from build123d import *

# Parameters (mm, degrees)
SKETCH1_W           = 78.9
SKETCH1_H           = 113.78
SKETCH1_R           = 2.75
BOSS_EXTRUDE1_DEPTH = 10
SKETCH2_R           = 11
CUT_EXTRUDE1_DEPTH  = 10
SKETCH3_R           = 22
CUT_EXTRUDE2_DEPTH  = 3
FILLET1_R           = 10


with BuildPart() as part:
    # Sketch1 → Boss-Extrude1 (new body)
    with BuildSketch(Plane(origin=(0, 0, 0), x_dir=(1, 0, 0), z_dir=(0, 1, 0))):
        with Locations((29.45, 46.89)):
            Rectangle(SKETCH1_W, SKETCH1_H)
        with Locations(Location((0, 93.78, 0), (0, 0, 270))):
            Circle(SKETCH1_R, mode=Mode.SUBTRACT)
        with Locations(Location((58.9, 93.78, 0), (0, 0, 270))):
            Circle(SKETCH1_R, mode=Mode.SUBTRACT)
        with Locations(Location((58.9, 0, 0), (0, 0, 270))):
            Circle(SKETCH1_R, mode=Mode.SUBTRACT)
        with Locations(Location((0, 0, 0), (0, 0, 270))):
            Circle(SKETCH1_R, mode=Mode.SUBTRACT)
        with Locations(Location((5.88, 70.46, 0), (0, 0, 270))):
            Circle(SKETCH1_R, mode=Mode.SUBTRACT)
        with Locations(Location((53.02, 70.46, 0), (0, 0, 270))):
            Circle(SKETCH1_R, mode=Mode.SUBTRACT)
        with Locations(Location((53.02, 23.32, 0), (0, 0, 270))):
            Circle(SKETCH1_R, mode=Mode.SUBTRACT)
        with Locations(Location((5.88, 23.32, 0), (0, 0, 270))):
            Circle(SKETCH1_R, mode=Mode.SUBTRACT)
    extrude(amount=BOSS_EXTRUDE1_DEPTH)

    # Sketch2 → Cut-Extrude1 (cut)
    with BuildSketch(Plane(origin=(0, 10, 0), x_dir=(1, 0, 0), z_dir=(0, 1, 0))):
        with Locations(Location((29.45, 46.89, 0), (0, 0, 270))):
            Circle(SKETCH2_R)
    extrude(amount=-CUT_EXTRUDE1_DEPTH, mode=Mode.SUBTRACT)

    # Sketch3 → Cut-Extrude2 (cut)
    with BuildSketch(Plane(origin=(0, 10, 0), x_dir=(1, 0, 0), z_dir=(0, 1, 0))):
        with Locations(Location((29.45, 46.89, 0), (0, 0, 270))):
            Circle(SKETCH3_R)
    extrude(amount=-CUT_EXTRUDE2_DEPTH, mode=Mode.SUBTRACT)

    # Fillet1
    fillet1_edges = [part.edges().sort_by_distance(p)[0] for p in [
        (-10, 5, 10),
        (-10, 5, -103.78),
        (68.9, 5, -103.78),
        (68.9, 5, 10),
    ]]
    fillet(fillet1_edges, radius=FILLET1_R)


solid = part.part
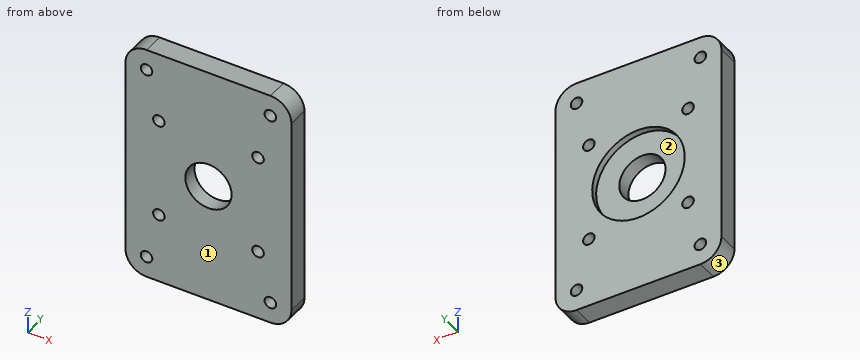
Design review of the part built by this model. Coordinates are the model's own, in mm. Face numbers are marked on the shaded views. Round coordinates to 2 decimals unless told otherwise and drop trailing zeros. Write each loop counter-clockwise with the first axis right and the second up, starting at its lowest first coordinate (ties: lowest second). Pieces come first, ordered by that corner, then holes. Notation, with made-up numbers: (-5, 16) - (33, 16) arc R15 cw to (33, 25) - close; hole circle Ø3 at (-22.75, 52). An arc over 180 degrees is marked (long way). Use a Markdown table: item, result. Add a question column.
1. We need section C-C (z = -46.89). State the section outline as (x, y) points.
2. Mouldability with a two-part tool opening along X and no side actions: class the marked faces 1, 2 and 3 as +X half, -X half, draft (parallel to the pull), parting line (faces both ways), or undercut.
3. We need section D-D (x = 29.45). State the section outline as (y, z) points.
4. We need section A-A (z = -23.32). State the section outline as (x, y) points.
5. Clearance check with a flat-ended pin moving along its axis: pin 1 (13 mm diameter, centred on x = 38.5, z = -50.5, fed in from +Y). State where the tip first meets the part, or that it passes through.
6. Wall thickness on probe 1 along X at (y, z) = (2, -23.32); probe 2 along X at (y, z) = (1.25, -92); probe 3 along Z at (x, y) = (8, 0.75): over which ranges is each line inside the solid? List them lowest first.
7. We need section B-B (x = 53.02). State the section outline as (y, z) points.
Output:
| question | item | result |
|---|---|---|
| 1 | outline | (-10, 0) - (18.45, 0) - (18.45, 7) - (7.45, 7) - (7.45, 10) - (-10, 10) - close; (40.45, 0) - (68.9, 0) - (68.9, 10) - (51.45, 10) - (51.45, 7) - (40.45, 7) - close |
| 2 | face 1 | draft |
| 2 | face 2 | undercut |
| 2 | face 3 | -X half |
| 3 | outline | (0, -103.78) - (10, -103.78) - (10, -68.89) - (7, -68.89) - (7, -57.89) - (0, -57.89) - close; (0, -35.89) - (7, -35.89) - (7, -24.89) - (10, -24.89) - (10, 10) - (0, 10) - close |
| 4 | outline | (-10, 0) - (3.13, 0) - (3.13, 10) - (-10, 10) - close; (8.63, 0) - (50.27, 0) - (50.27, 10) - (8.63, 10) - close; (55.77, 0) - (68.9, 0) - (68.9, 10) - (55.77, 10) - close |
| 5 | pin 1 | stops at y = 7 |
| 6 | probe 1 | x = -10 to 3.13, 8.63 to 50.27, 55.77 to 68.9 |
| 6 | probe 2 | x = -10 to -2.1, 2.1 to 56.8, 61 to 68.9 |
| 6 | probe 3 | z = -103.78 to -72.21, -68.71 to -25.07, -21.57 to 10 |
| 7 | outline | (0, -103.78) - (10, -103.78) - (10, -73.21) - (0, -73.21) - close; (0, -67.71) - (10, -67.71) - (10, -26.07) - (0, -26.07) - close; (0, -20.57) - (10, -20.57) - (10, 10) - (0, 10) - close |
